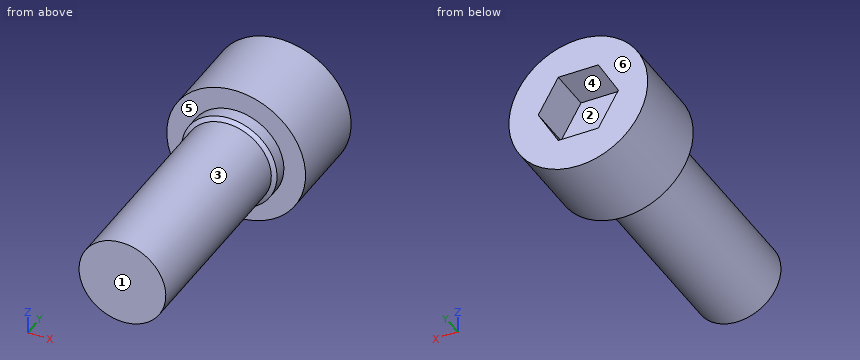
```python
from build123d import *

# Parameters (mm, degrees)
CUT_EXTRUDE1_DEPTH = 5


with BuildPart() as part:
    # Sketch1 → Revolve1 (revolve)
    with BuildSketch(Plane.XY, mode=Mode.PRIVATE) as revolve1_sk:
        Polygon((0, -25), (5, -25), (5, 0), (8, 0), (8, 10), (0, 10), align=None)
    revolve(revolve1_sk.sketch.rotate(Axis((0, 61.691642626, 0), (0, -1, 0)), 90), axis=Axis((0, 61.691642626, 0), (0, -1, 0)))

    # Sketch2 → Cut-Extrude1 (cut)
    with BuildSketch(Plane(origin=(0, 10, 0), x_dir=(-1, 0, 0), z_dir=(0, 1, 0))):
        Polygon((-2.309401077, -4), (2.309401077, -4), (4.618802154, 0), (2.309401077, 4), (-2.309401077, 4), (-4.618802154, 0), align=None)
    extrude(amount=-CUT_EXTRUDE1_DEPTH, mode=Mode.SUBTRACT)

    # Sketch3 → O-ring relief in hole (revolve)
    with BuildSketch(Plane.XY, mode=Mode.PRIVATE) as o_ring_relief_in_hole_sk:
        Polygon((0, 0), (5.5, 0), (5.5, -1.5), (0, -4.936781436), align=None)
    revolve(o_ring_relief_in_hole_sk.sketch.rotate(Axis((0, 0, 0), (0, -1, 0)), 90), axis=Axis((0, 0, 0), (0, -1, 0)))


solid = part.part
```
Part model, mm, in its own coordinate system. Face numbers are marked on the shaded views. A direction names the side the tool comes from. Round coordinates to 2 decimals unless told otherwise and drop trailing zeros. Loops run counter-clockwise (first coordinate to the right, second up) from the corner with the lowest first, then second, coordinate; pieces in that order, holes last.
1. Drill centre lines: line 1 along Y through (x, z) = (-6, -2.25); line 2 along Y through (x, z) = (-3.5, -0.25); line 3 along X through (y, z) = (-22, -0.25). Where is each one in solid material? Low to high.
Solutions:
line 1: y = 0 to 10
line 2: y = -25 to 5
line 3: x = -4.99 to 4.99
2. Flat gauge pins, fed straight in: pin 1 (1 mm diameter, centred on x = 1, y = -7, fed in from +Z); pin 2 (4 mm diameter, centred on x = 1.5, y = -6, fed in from -Z); pin 3 (2 mm diameter, centred on y = -19, z = 0.5, fed in from -X). Where does each tip first touch, or does it go through?
Solutions:
pin 1: stops at z = 4.97
pin 2: stops at z = -5
pin 3: stops at x = -5
3. 3-axis set-ups, long thin cutter, end or side, ignore diameter. For the marked faces 4, 5 and 6: which of +Z, -Z, +X, -X, +Y, -Y reach the whole face in a straight line?
Solutions:
face 4: +Y
face 5: -Y
face 6: +Z, -Z, +X, -X, +Y
4. Two-plate mould, pull along X, no slides. Class the marked faces 1, 2 and 3: pulls with the +X half, pulls with the -X half, needs draft (parallel to the pull), parting line crosses it, or undercut.
Solutions:
face 1: needs draft
face 2: undercut
face 3: parting line crosses it
5. Slice it at C-C (y = 0.5). Give the cut face in (x, z), and give its area (3 significant figures).
Solutions:
outline: circle Ø16 at (0, 0)
area: 201 mm2
6. Slice it at B-B (y = -8.5). Give the cut face in (x, z), and give its area (3 significant figures).
Solutions:
outline: circle Ø10 at (0, 0)
area: 78.5 mm2
7. Slice it at A-A (x = 0). Give the cut face in (y, z), and give its area (3 significant figures).
Solutions:
outline: (-25, -5) - (-1.81, -5) - (-1.5, -5.5) - (0, -5.5) - (0, -8) - (10, -8) - (10, -4) - (5, -4) - (5, 4) - (10, 4) - (10, 8) - (0, 8) - (0, 5.5) - (-1.5, 5.5) - (-1.81, 5) - (-25, 5) - close
area: 372 mm2
